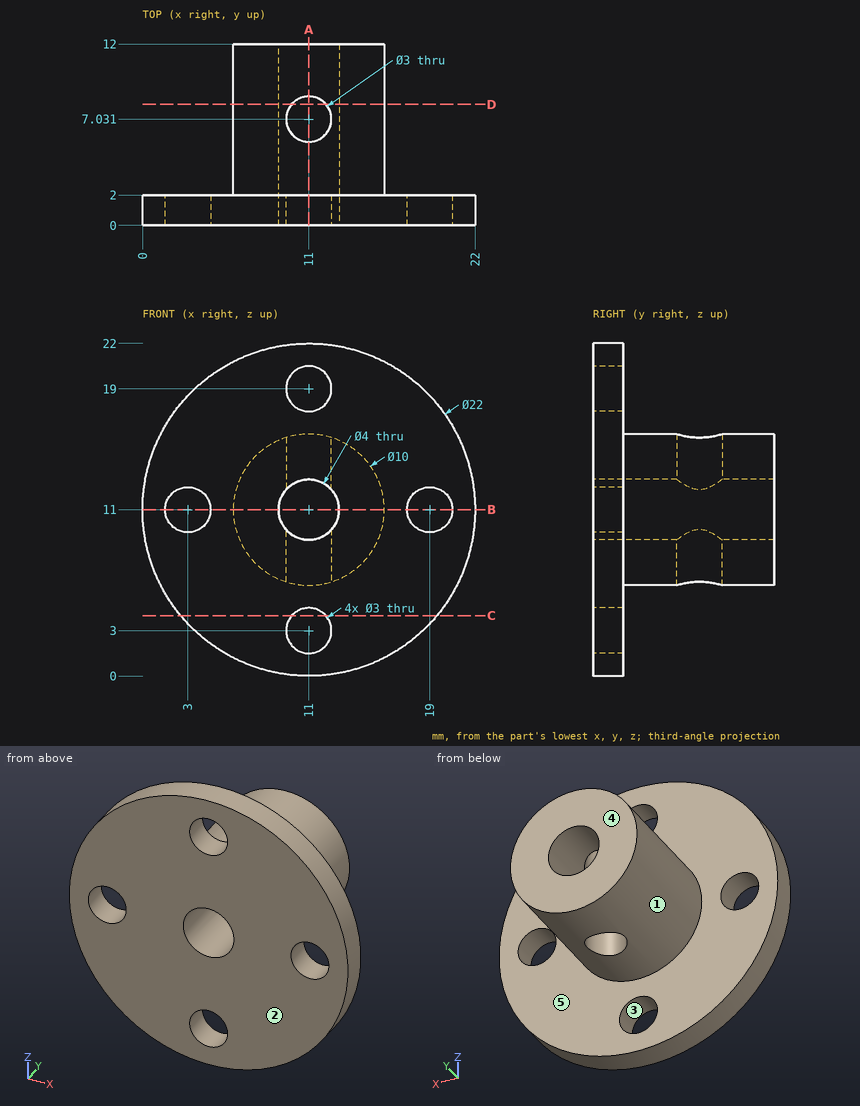
Could you check a few things on this drawing? It's one solid part, dimensions in mm from its lowest x, y, z. A direction names the side the tool comes from. Round coordinates to 2 decimals unless told otherwise and drop trailing zeros. Order: outer loops, then holes, each group sorted by start corner. A loop starts at its lowest first (then second) coordinate and runs counter-clockwise, first axis right, second up.
Q1. Imagine slicing it at D-D, the plane y = 8. List the corners of the cut face in (x, z) for me (1 decimal), then the cut area to 3 significant figures.
Geometry says:
outline: (9.9, 6.1) - (9.9, 9.4) arc R2 cw to (9.9, 12.6) - (9.9, 15.9) arc R5 ccw to start; (12.1, 6.1) arc R5 ccw to (12.1, 15.9) - (12.1, 12.6) arc R2 cw to (12.1, 9.4) - close
area: 51.9 mm2
Q2. Imagine slicing it at B-B, the plane z = 11. List the corners of the cut face in (x, y) for me.
Geometry says:
outline: (0, 0) - (1.5, 0) - (1.5, 2) - (0, 2) - close; (4.5, 0) - (9, 0) - (9, 12) - (6, 12) - (6, 2) - (4.5, 2) - close; (13, 0) - (17.5, 0) - (17.5, 2) - (16, 2) - (16, 12) - (13, 12) - close; (20.5, 0) - (22, 0) - (22, 2) - (20.5, 2) - close
Q3. Thinking about a two-plate mould opening in Z: for the marked faces 1, 2 and 3, which applies, released by +Z, released by -Z, zero draft, split by the parting line, or undercut?
Geometry says:
face 1: split by the parting line
face 2: zero draft
face 3: undercut
Q4. Which directions (+Z, -Z, +X, -X, +Y, -Y) give clear straight access to the entire face, cutting with the end or side of a thin tool? Please do the marked faces 4 and 5.
Geometry says:
face 4: +Z, -Z, +X, -X, +Y
face 5: +Y
Q5. Imagine slicing it at A-A, the plane x = 11. List the corners of the cut face in (y, z) for me.
Geometry says:
outline: (0, 0) - (2, 0) - (2, 1.5) - (0, 1.5) - close; (0, 4.5) - (2, 4.5) - (2, 6) - (5.53, 6) - (5.53, 9) - (0, 9) - close; (0, 13) - (5.53, 13) - (5.53, 16) - (2, 16) - (2, 17.5) - (0, 17.5) - close; (0, 20.5) - (2, 20.5) - (2, 22) - (0, 22) - close; (8.53, 6) - (12, 6) - (12, 9) - (8.53, 9) - close; (8.53, 13) - (12, 13) - (12, 16) - (8.53, 16) - close
Q6. Please list where these lines run through material, in increasing order: probe 1 along Z at (x, y) = (11, 1); probe 2 along Y at (x, z) = (11, 14.3); probe 3 along Z at (x, y) = (11, 3.5).
Geometry says:
probe 1: z = 0 to 1.5, 4.5 to 9, 13 to 17.5, 20.5 to 22
probe 2: y = 0 to 5.53, 8.53 to 12
probe 3: z = 6 to 9, 13 to 16
Q7. Imagine slicing it at C-C, the plane z = 4. List the corners of the cut face in (x, y) for me (1 decimal).
Geometry says:
outline: (2.5, 0) - (9.9, 0) - (9.9, 2) - (2.5, 2) - close; (12.1, 0) - (19.5, 0) - (19.5, 2) - (12.1, 2) - close
Q8. I'm going to push flat-ended pins straight in: P1, Ø2.5, axis at x = 11, y = 7.03, coming from the -Z side; P2, Ø3, axis at x = 14.5, y = 6.5, coming from the +Z side; P3, Ø1, axis at x = 18.5, z = 15, coming from the +Y side; P4, Ø3, axis at y = 3, z = 13, coming from the -X side (1 decimal). Where does each tip first touch, or does it pass through?
Geometry says:
P1: passes through
P2: stops at z = 15.58
P3: stops at y = 2
P4: stops at x = 0
